```python
from build123d import *

# Parameters (mm, degrees)
SKETCH1_R           = 1.5
BOSS_EXTRUDE1_DEPTH = 3
SKETCH2_W           = 40
SKETCH2_H           = 3
SKETCH2_W_2         = 3
SKETCH2_H_2         = 36
SKETCH2_H_3         = 40
SKETCH2_W_3         = 35
SKETCH2_W_4         = 30
SKETCH2_H_4         = 35
CUT_EXTRUDE1_DEPTH  = 3


with BuildPart() as part:
    # Sketch1 → Boss-Extrude1 (new body)
    with BuildSketch(Plane.XY.offset(-1194.952985965)):
        with BuildLine():
            ThreePointArc((-135, 1558.280393103), (-147.632217989, 1553.786103944), (-154.587151942, 1542.323099971))
            Line((-154.587151942, 1542.323099971), (-176.967879854, 1433.887160273))
            ThreePointArc((-176.967879854, 1433.887160273), (-177.74130071, 1428.860058806), (-178, 1423.780393103))
            Line((-178, 1423.780393103), (-178, 1292.280393103))
            ThreePointArc((-178, 1292.280393103), (-175.071067812, 1285.209325291), (-168, 1282.280393103))
            Line((-168, 1282.280393103), (-163, 1282.280393103))
            Line((-163, 1282.280393103), (-163, 1196.280393103))
            Line((-163, 1196.280393103), (-168, 1196.280393103))
            ThreePointArc((-168, 1196.280393103), (-175.071067812, 1193.351460915), (-178, 1186.280393103))
            Line((-178, 1186.280393103), (-178, 1165.280393103))
            ThreePointArc((-178, 1165.280393103), (-175.071067812, 1158.209325291), (-168, 1155.280393103))
            Line((-168, 1155.280393103), (168, 1155.280393103))
            ThreePointArc((168, 1155.280393103), (175.071067812, 1158.209325291), (178, 1165.280393103))
            Line((178, 1165.280393103), (178, 1423.782857009))
            ThreePointArc((178, 1423.782857009), (177.70399808, 1429.215404737), (176.819497007, 1434.583630683))
            Line((176.819497007, 1434.583630683), (152.921914731, 1542.600702573))
            ThreePointArc((152.921914731, 1542.600702573), (145.915973031, 1553.875363276), (133.394115928, 1558.280393103))
            Line((133.394115928, 1558.280393103), (-135, 1558.280393103))
        make_face()
        with Locations((-171, 1176.280393103)):
            Circle(SKETCH1_R, mode=Mode.SUBTRACT)
        with Locations((-128, 1161.280393103)):
            Circle(SKETCH1_R, mode=Mode.SUBTRACT)
        with Locations((-43, 1161.280393103)):
            Circle(SKETCH1_R, mode=Mode.SUBTRACT)
        with Locations((-171, 1302.280393103)):
            Circle(SKETCH1_R, mode=Mode.SUBTRACT)
        with Locations((43, 1161.280393103)):
            Circle(SKETCH1_R, mode=Mode.SUBTRACT)
        with Locations((128, 1161.280393103)):
            Circle(SKETCH1_R, mode=Mode.SUBTRACT)
        with Locations((171, 1217.280393103)):
            Circle(SKETCH1_R, mode=Mode.SUBTRACT)
        with Locations((171, 1297.280393103)):
            Circle(SKETCH1_R, mode=Mode.SUBTRACT)
        with Locations((-171, 1382.280393103)):
            Circle(SKETCH1_R, mode=Mode.SUBTRACT)
        with Locations((-164.628822574, 1457.280393103)):
            Circle(SKETCH1_R, mode=Mode.SUBTRACT)
        with Locations((-151.667894165, 1515.863789512)):
            Circle(SKETCH1_R, mode=Mode.SUBTRACT)
        with Locations((-104.587151942, 1551.280393103)):
            Circle(SKETCH1_R, mode=Mode.SUBTRACT)
        with Locations((-34.587151942, 1551.280393103)):
            Circle(SKETCH1_R, mode=Mode.SUBTRACT)
        Polygon((160, 1173.280393103), (-160, 1173.280393103), (-160, 1282.280393103), (-160, 1427.280393103), (-135, 1540.280393103), (135, 1540.280393103), (160, 1427.280393103), align=None, mode=Mode.SUBTRACT)
        with Locations((171, 1377.280393103)):
            Circle(SKETCH1_R, mode=Mode.SUBTRACT)
        with Locations((164.628822573, 1457.280393103)):
            Circle(SKETCH1_R, mode=Mode.SUBTRACT)
        with Locations((32.921914731, 1551.280393103)):
            Circle(SKETCH1_R, mode=Mode.SUBTRACT)
        with Locations((102.921914731, 1551.280393103)):
            Circle(SKETCH1_R, mode=Mode.SUBTRACT)
        with Locations((151.667894164, 1515.863789512)):
            Circle(SKETCH1_R, mode=Mode.SUBTRACT)
    extrude(amount=BOSS_EXTRUDE1_DEPTH)

    # Sketch2 → Cut-Extrude1 (cut)
    with BuildSketch(Plane.XY.offset(-1191.952985965)):
        with Locations((-118, 1171.780393103)):
            Rectangle(SKETCH2_W, SKETCH2_H)
        with Locations((-38, 1171.780393103)):
            Rectangle(SKETCH2_W, SKETCH2_H)
        with Locations((42, 1171.780393103)):
            Rectangle(SKETCH2_W, SKETCH2_H)
        with Locations((122, 1171.780393103)):
            Rectangle(SKETCH2_W, SKETCH2_H)
        with Locations((-161.5, 1239.280393103)):
            Rectangle(SKETCH2_W_2, SKETCH2_H_2)
        with Locations((-161.5, 1317.280393103)):
            Rectangle(SKETCH2_W_2, SKETCH2_H_3)
        with Locations((-161.5, 1397.280393103)):
            Rectangle(SKETCH2_W_2, SKETCH2_H_3)
        with Locations((-87.5, 1541.780393103)):
            Rectangle(SKETCH2_W_3, SKETCH2_H)
        with Locations((-20, 1541.780393103)):
            Rectangle(SKETCH2_W_4, SKETCH2_H)
        with Locations((35, 1541.780393103)):
            Rectangle(SKETCH2_W_4, SKETCH2_H)
        with Locations((90, 1541.780393103)):
            Rectangle(SKETCH2_W_4, SKETCH2_H)
        with Locations((161.5, 1295.780393103)):
            Rectangle(SKETCH2_W_2, SKETCH2_H_4)
        with Locations((161.5, 1210.780393103)):
            Rectangle(SKETCH2_W_2, SKETCH2_H_4)
        with Locations((161.5, 1365.780393103)):
            Rectangle(SKETCH2_W_2, SKETCH2_H_4)
    extrude(amount=-CUT_EXTRUDE1_DEPTH, mode=Mode.SUBTRACT)


solid = part.part
```
Here's how the part is built. I have some questions about the finished solid (model axes, mm). A direction names the side the tool comes from. Round coordinates to 2 decimals unless told otherwise and drop trailing zeros. Loops run counter-clockwise (first coordinate to the right, second up) from the corner with the lowest first, then second, coordinate; pieces in that order, holes last. Notation, with made-up numbers: (68.25, -7.75) -> (79.25, -7.75) arc R3 ccw to (79.25, -2.75) -> close; hole circle Ø1 at (-3, 27). An arc over 180 degrees is marked (long way). Answer as CSV lines item,"result". Start each with the question number.
1. If we mould it in two halves opening along X, with no side actions, what happens to faces 1 (the face through (171, 1373, -1191.953)), 2 (the face through (146.06, 1553.76, -1193.47)), 3 (the face through (-147.675, 1482.989, -1193.474))? For each: pulls with the +X half, pulls with the -X half, needs draft (parallel to the pull), parting line crosses it, or undercut.
2. Imagine slicing it at B-B on x = 80. Write out the boundary of the cut face in (y, z), plus the area to 3 significant figures.
3. I need wall thicknesses on probe 1 along Y at (x, z) = (43, -1193.9); probe 2 along X at (y, z) = (1395.5, -1194.1); probe 3 along Y at (x, z) = (-62, -1192.85). Which ranges of each line are inside material? Lowest first, please. Write a range as from..to.
4. Imagine slicing it at A-A on y = 1363. Write out the boundary of the cut face in (x, z), plus the area to 3 significant figures.
5. For faces 4 (the face through (165, 1488, -1193)), 5 (the face through (-174.99, 1193.43, -1193.47)), 6 (the face through (147.325, 1484.571, -1193.474)), which set-ups out of +Z, -Z, +X, -X, +Y, -Y let a thin tool reach every point of the face, with its end or its side?
6. Imagine slicing it at C-C on z = -1193.2. State how many separate pieces and enclosed holes the cut face has, plus the area to 3 significant figures.
7. I'm going to push flat-ended pins straight in: P1, Ø0.9, axis at y = 1215, z = -1194, coming from the -X side; P2, Ø1, axis at y = 1425.5, z = -1192.5, coming from the +X side; P3, Ø1.5, axis at y = 1542, z = -1193.5, coming from the -X side. Where does each tip first touch, or does it pass through?
Solution:
1,face 1,"needs draft"
1,face 2,"pulls with the +X half"
1,face 3,"undercut"
2,outline,"(1155.28, -1194.95) -> (1173.28, -1194.95) -> (1173.28, -1191.95) -> (1155.28, -1191.95) -> close; (1543.28, -1194.95) -> (1558.28, -1194.95) -> (1558.28, -1191.95) -> (1543.28, -1191.95) -> close"
2,area,"99.0 mm²"
3,probe 1,"1155.28..1159.78, 1162.78..1170.28, 1543.28..1558.28"
3,probe 2,"-178..-163, 160..178"
3,probe 3,"1155.28..1173.28, 1540.28..1558.28"
4,outline,"(-178, -1194.95) -> (-160, -1194.95) -> (-160, -1191.95) -> (-178, -1191.95) -> close; (163, -1194.95) -> (178, -1194.95) -> (178, -1191.95) -> (163, -1191.95) -> close"
4,area,"99.0 mm²"
5,face 4,"+Z, -Z, +X, +Y"
5,face 5,"+Z, -Z, -X"
5,face 6,"+Z, -Z"
6,separate pieces,"1"
6,enclosed holes,"18"
6,area,"22,200 mm²"
7,P1,"x = -163"
7,P2,"x = 177.99"
7,P3,"x = -154.81"
